Check sheet for the modelled part. Datum: model origin and axes. Units: mm. A direction names the side the tool comes from. Coordinates: 2 decimals unless noted, no trailing zeros. Write each loop counter-clockwise with the first axis right and the second up, starting at its lowest first coordinate (ties: lowest second). Pieces come first, ordered by that corner, then holes. Notation, with made-up numbers: M -2.75,56 L 29.25,56 A5 cw 29.25,62 Z; hole C -37,57 d4. An arc over 180 degrees is marked long. Answer as CSV lines item,"result". Start each with the question number.
1) Section check D-D (z = -33). Record the cut outline in (x, y).
2) Access from +Z, -Z, +X, -X, +Y, -Y to the whole of each face (thin tool, end or side, straight path). Record for faces 1 (the flat face through (-1, 119, 29.76)), 2 (the flat face through (0, 200, 2)), 3 (the cylindrical face through (2.24, 118.88, -24.9)).
3) Section check A-A (z = 0). Record the cut outline in (x, y), and give its area (3 significant figures).
4) Go/stop test with flat-tipped pins: pin 1 Ø2 at (x, z) = (41, 95.5) entering from +Y; pin 2 Ø2.5 at (y, z) = (145.5, 26.5) entering from -X; pin 3 Ø7.5 at (x, y) = (-1, 149) entering from +Z. Record where each tip stops, or that it passes through.
5) Section check B-B (x = 7.5). Record the cut outline in (y, z).
6) Section check C-C (y = 92). Record the cut outline in (x, z).
7) Material ranges on L1, parallel to Y at x = -94, z = 114; L2, parallel to X at y = 135.5, z = 26; L3, parallel to Z at x = -133.5, y = 17, recorded low to high. Write a range as [from, to].
from build123d import *

# Parameters (mm, degrees)
SKETCH1_R           = 150
BOSS_EXTRUDE1_DEPTH = 40
BOSS_EXTRUDE2_DEPTH = 200


with BuildPart() as part:
    # Sketch1 → Boss-Extrude1 (new body)
    with BuildSketch(Plane(origin=(0, 0, 0), x_dir=(1, 0, 0), z_dir=(0, 1, 0))):
        with Locations(Location((0, 0, 0), (0, 0, 270))):
            Circle(SKETCH1_R)
        with BuildLine():
            Line((-5.790928426, -29.760056496), (-5.790928426, -24.320056496))
            ThreePointArc((-5.790928426, -24.320056496), (-15.49559275, 19.618527094), (25, 0))
            ThreePointArc((25, 0), (18.844452623, -16.428225873), (3.409071574, -24.766473932))
            Line((3.409071574, -24.766473932), (3.409071574, -29.760056496))
            Line((3.409071574, -29.760056496), (-5.790928426, -29.760056496))
        make_face(mode=Mode.SUBTRACT)
    extrude(amount=BOSS_EXTRUDE1_DEPTH)

    # Sketch1_3 → Boss-Extrude2 (add)
    with BuildSketch(Plane(origin=(0, 0, 0), x_dir=(1, 0, 0), z_dir=(0, 1, 0))):
        with BuildLine():
            ThreePointArc((3.409071574, -24.766473932), (1.211665237, 24.970620083), (-5.790928426, -24.320056496))
            Line((-5.790928426, -24.320056496), (-5.790928426, -29.760056496))
            Line((-5.790928426, -29.760056496), (3.409071574, -29.760056496))
            Line((3.409071574, -29.760056496), (3.409071574, -24.766473932))
        make_face()
    extrude(amount=BOSS_EXTRUDE2_DEPTH)


solid = part.part
Results found:
1,outline,"M -146.32,0 L 146.32,0 L 146.32,40 L -146.32,40 Z"
2,face 1,"+Z, +X, -X, +Y"
2,face 2,"+Z, -Z, +X, -X, +Y"
2,face 3,"+Y"
3,outline,"M -150,0 L 150,0 L 150,40 L 25,40 L 25,200 L -25,200 L -25,40 L -150,40 Z"
3,area,"20,000 mm2"
4,pin 1,"stops at y = 40"
4,pin 2,"stops at x = -5.79"
4,pin 3,"stops at z = 29.76"
5,outline,"M 0,-149.81 L 40,-149.81 L 40,-23.85 L 200,-23.85 L 200,23.85 L 40,23.85 L 40,149.81 L 0,149.81 Z"
6,outline,"M -5.79,24.32 A25 ccw long 3.41,24.77 L 3.41,29.76 L -5.79,29.76 Z"
7,L1,"y = [0, 40]"
7,L2,"x = [-5.79, 3.41]"
7,L3,"z = [-68.39, 68.39]"
